Geometry: final body of the model. Coordinates: model frame, mm. A direction names the side the tool comes from. Give positions to 0.01 mm unless a question says otherwise; leave off trailing zeros. Write each loop counter-clockwise with the first axis right and the second up, starting at its lowest first coordinate (ties: lowest second). Pieces come first, ordered by that corner, then holes. Notation, with made-up numbers: (44, 70.25) -> (95, 70.25) arc R32 cw to (95, 106.25) -> close; hole circle Ø3 at (21.5, 81). An arc over 180 degrees is marked (long way). Answer as a JSON object with one key per item and string values.
from build123d import *
from build123d.topology import SkipClean

# Parameters (mm, degrees)
BOSS_EXTRUDE1_DEPTH             = 25
BOSS_EXTRUDE2_REACH             = 65.362
BOSS_EXTRUDE2_DIRECTION_2_DEPTH = 30
SKETCH9_R                       = 2.05
CUT_EXTRUDE3_DEPTH              = 35
BOSS_EXTRUDE5_REACH             = 62.896
SKETCH13_R                      = 1.55
CUT_EXTRUDE4_DEPTH              = 87.254538717
SKETCH16_W                      = 50
SKETCH16_H                      = 45
CUT_EXTRUDE5_DEPTH              = 17.5
BOSS_EXTRUDE6_DEPTH             = 17.5
SKETCH20_R                      = 2.05
CUT_EXTRUDE6_DEPTH              = 17.5


with BuildPart() as part:
    # Sketch1 → Boss-Extrude1 (new, symmetric)
    with BuildSketch(Plane.XY):
        with BuildLine():
            Line((-17.5, 22.5), (-17.5, 0))
            Line((-17.5, 0), (17.5, 0))
            Line((17.5, 0), (17.5, 22.5))
            Line((17.5, 22.5), (12.5, 22.5))
            ThreePointArc((12.5, 22.5), (0, 10), (-12.5, 22.5))
            Line((-12.5, 22.5), (-17.5, 22.5))
        make_face()
    boss_extrude1 = extrude(amount=BOSS_EXTRUDE1_DEPTH, both=True)

    # Boss-Extrude2: up to this face of the body (flat: up to its plane)
    boss_extrude2_end = Plane(part.part.faces().sort_by_distance((17.5, 11.25, 0))[0])
    # Sketch5 → Boss-Extrude2 (add, up to the picked face)
    with BuildSketch(Plane(origin=(26.115381057, 0, 15.077722283), x_dir=(0.500000000000001, 0, -0.8660254037844382), z_dir=(0.8660254037844382, 0, 0.500000000000001)), mode=Mode.PRIVATE) as boss_extrude2_sk1:
        with BuildLine():
            Line((-6.75, 22.5), (-3.9, 22.5))
            ThreePointArc((-3.9, 22.5), (8.75, 9.85), (21.4, 22.5))
            Line((21.4, 22.5), (24.25, 22.5))
            ThreePointArc((24.25, 22.5), (8.75, 7), (-6.75, 22.5))
        make_face()
    boss_extrude2_tool1 = split(extrude(boss_extrude2_sk1.sketch, amount=-BOSS_EXTRUDE2_REACH, mode=Mode.PRIVATE), bisect_by=boss_extrude2_end, keep=Keep.BOTH, mode=Mode.PRIVATE)
    boss_extrude2 = boss_extrude2_tool1.solids().sort_by(Axis((23.452881, 22.153409, 19.689308), (-0.8660254037844382, 0, -0.500000000000001)))[0]
    add(boss_extrude2)

    # Sketch5 → Boss-Extrude2 direction 2 (add)
    with BuildSketch(Plane(origin=(26.115381057, 0, 15.077722283), x_dir=(0.500000000000001, 0, -0.8660254037844382), z_dir=(0.8660254037844382, 0, 0.500000000000001))):
        with BuildLine():
            Line((-6.75, 22.5), (-3.9, 22.5))
            ThreePointArc((-3.9, 22.5), (8.75, 9.85), (21.4, 22.5))
            Line((21.4, 22.5), (24.25, 22.5))
            ThreePointArc((24.25, 22.5), (8.75, 7), (-6.75, 22.5))
        make_face()
    boss_extrude2_direction_2 = extrude(amount=BOSS_EXTRUDE2_DIRECTION_2_DEPTH)

    # Sketch9 → Cut-Extrude3 (cut)
    with BuildSketch(Plane.ZY.offset(17.5)):
        with Locations((-18, 5)):
            Circle(SKETCH9_R)
    cut_extrude3 = extrude(amount=-CUT_EXTRUDE3_DEPTH, mode=Mode.SUBTRACT)

    # Boss-Extrude5: up to this face of the body (flat: up to its plane)
    boss_extrude5_end = Plane(part.part.faces().sort_by_distance((17.5, 17.131173253, 0))[0])
    # Sketch12 → Boss-Extrude5 (add, up to the picked face)
    with BuildSketch(Plane(origin=(22.048076211, 0, 12.729462736), x_dir=(0.4999999999999999, 0, -0.8660254037844388), z_dir=(0.8660254037844388, 0, 0.4999999999999999)), mode=Mode.PRIVATE) as boss_extrude5_sk1:
        with BuildLine():
            Line((-3.9, 22.5), (21.4, 22.5))
            ThreePointArc((21.4, 22.5), (8.75, 9.85), (-3.9, 22.5))
        make_face()
    boss_extrude5_tool1 = split(extrude(boss_extrude5_sk1.sketch, amount=-BOSS_EXTRUDE5_REACH, mode=Mode.PRIVATE), bisect_by=boss_extrude5_end, keep=Keep.BOTH, mode=Mode.PRIVATE)
    boss_extrude5 = boss_extrude5_tool1.solids().sort_by(Axis((26.423076, 17.131173, 5.15174), (-0.8660254037844388, 0, -0.4999999999999999)))[0]
    add(boss_extrude5)

    # Mirror1: Boss-Extrude1, Boss-Extrude2, Boss-Extrude2 direction 2, Cut-Extrude3, Boss-Extrude5 across plane
    with SkipClean():  # the faces are left unmerged after this step: merging them gives an invalid solid
        add(boss_extrude1.mirror(Plane(origin=(17.5, 22.5, 25), x_dir=(0, 0, 1), z_dir=(0, -1, 0))))
        add(boss_extrude2.mirror(Plane(origin=(17.5, 22.5, 25), x_dir=(0, 0, 1), z_dir=(0, -1, 0))))
        add(boss_extrude2_direction_2.mirror(Plane(origin=(17.5, 22.5, 25), x_dir=(0, 0, 1), z_dir=(0, -1, 0))))
        add(cut_extrude3.mirror(Plane(origin=(17.5, 22.5, 25), x_dir=(0, 0, 1), z_dir=(0, -1, 0))), mode=Mode.SUBTRACT)
        add(boss_extrude5.mirror(Plane(origin=(17.5, 22.5, 25), x_dir=(0, 0, 1), z_dir=(0, -1, 0))))

    # Sketch13 → Cut-Extrude4 (cut, through all)
    with SkipClean():  # the faces are left unmerged after this step: merging them gives an invalid solid
        with BuildSketch(Plane(origin=(0, 0, 0), x_dir=(1, 0, 0), z_dir=(0, 1, 0))):
            with Locations(Location((43.480762114, -15, 0), (0, 0, 90))):
                Circle(SKETCH13_R)
        extrude(amount=CUT_EXTRUDE4_DEPTH, mode=Mode.SUBTRACT)

    # Sketch16 → Cut-Extrude5 (cut)
    with SkipClean():  # the faces are left unmerged after this step: merging them gives an invalid solid
        with BuildSketch(Plane(origin=(0, 0, 0), x_dir=(0, 0, -1), z_dir=(1, 0, 0))):
            with Locations((0, 22.5)):
                Rectangle(SKETCH16_W, SKETCH16_H)
        extrude(amount=-CUT_EXTRUDE5_DEPTH, mode=Mode.SUBTRACT)
    add(part.part.scale(1), mode=Mode.REPLACE)  # the faces are merged on a copy

    # Sketch18 → Boss-Extrude6 (add)
    with BuildSketch(Plane.ZY):
        with BuildLine():
            Line((13, 0), (23, 0))
            ThreePointArc((23, 0), (18, -5), (13, 0))
        make_face()
    boss_extrude6 = extrude(amount=-BOSS_EXTRUDE6_DEPTH)

    # Sketch20 → Cut-Extrude6 (cut)
    with BuildSketch(Plane.ZY):
        with Locations((18, 0)):
            Circle(SKETCH20_R)
    cut_extrude6 = extrude(amount=-CUT_EXTRUDE6_DEPTH, mode=Mode.SUBTRACT)

    # Mirror2: Boss-Extrude6, Cut-Extrude6 across plane
    add(boss_extrude6.mirror(Plane.ZX.offset(22.5)))
    add(cut_extrude6.mirror(Plane.ZX.offset(22.5)), mode=Mode.SUBTRACT)


solid = part.part
Q1. Set-up query: faces 4 (the flat face through (9, 0, -6)), 5 (the flat face through (9, 0, 24)), 6 (the flat face through (26.51, 22.32, 5)), 7 (the flat face through (9, 45, -6)). Return all of +Z, -Z, +X, -X, +Y, -Y with unobstructed straight access to the full face (end or side cutting, diameter ignored); none if empty.
Values:
{"face 4": "-Z, +X, -X, -Y", "face 5": "+Z, +X, -X, -Y", "face 6": "none", "face 7": "-Z, +X, -X, +Y"}
Q2. Mould query, pull axis Z, two halves, no side actions, for faces 1 (the cylindrical face through (44.424, 36.506, 16.23)), 2 (the flat face through (59.378, 11.091, 17.466)), 3 (the flat face through (9, 45, 24)). Classes: pulls with the +Z half, pulls with the -Z half, needs draft (parallel to the pull), parting line crosses it, or undercut.
Values:
{"face 1": "undercut", "face 2": "pulls with the +Z half", "face 3": "needs draft"}
Q3. First-contact query: P1, Ø4, axis at y = 47, z = 18, coming from the +X side; P2, Ø6, axis at x = 17.5, z = 24, coming from the +Y side; P3, Ø3.5, axis at y = 45, z = 18, coming from the -X side; P4, Ø9, axis at x = 6.5, y = 17, coming from the +Z side. Flat tips, straight axial feed; report the tip coordinate or a pass-through.
Values:
{"P1": "x = 17.5", "P2": "y = 49", "P3": "through", "P4": "z = 25"}
Q4. Cut plane B-B (z = 15). State how many separate pieces and enclosed holes the cut face has, and give its area (3 significant figures).
Values:
{"separate pieces": "3", "enclosed holes": "0", "area": "984 mm²"}
Q5. Cut plane A-A (y = 5). Return the cut outline in (x, z), and give its area (3 significant figures).
Values:
{"outline": "(0, -25) -> (17.5, -25) -> (17.5, -20.05) -> (0, -20.05) -> close; (0, -15.95) -> (17.5, -15.95) -> (17.5, 25) -> (0, 25) -> close", "area": "803 mm²"}
Q6. Material intervals for L1, parallel to Y at x = 14.25, z = -18; L2, parallel to Z at x = 12.75, y = 40; L3, parallel to Y at x = 40, z = 13, sorted ascending. Write a range as from..to.
Values:
{"L1": "0..2.95, 7.05..37.95, 42.05..45", "L2": "-25..-20.05, -15.95..25", "L3": "7..9.85, 35.15..38"}
